Check sheet for the modelled part. Datum: model origin and axes. Units: mm. Face numbers are marked on the shaded views. A direction names the side the tool comes from. Round coordinates to 2 decimals unless told otherwise and drop trailing zeros. Write each loop counter-clockwise with the first axis right and the second up, starting at its lowest first coordinate (ties: lowest second). Pieces come first, ordered by that corner, then holes. Notation, with made-up numbers: M -33.75,89 L 18.25,89 A33 ccw 18.25,128 Z; hole C 32,24.5 d5. An arc over 180 degrees is marked long. One line per item, written item: value.
from build123d import *

# Parameters (mm, degrees)
ESQUISSE1_W        = 6
ESQUISSE1_H        = 55
BOSS_EXTRU_1_DEPTH = 3.5
ESQUISSE2_W        = 6
ESQUISSE2_H        = 2.5
BOSS_EXTRU_2_DEPTH = 35
ESQUISSE4_W        = 6
ESQUISSE4_H        = 2
BOSS_EXTRU_3_DEPTH = 15
ESQUISSE10_R       = 2.25
BOSS_EXTRU_4_DEPTH = 4.7
CONG_5_R           = 1


with BuildPart() as part:
    # Esquisse1 → Boss.-Extru.1 (new body)
    with BuildSketch(Plane.XY):
        with Locations((3, 27.5)):
            Rectangle(ESQUISSE1_W, ESQUISSE1_H)
    extrude(amount=BOSS_EXTRU_1_DEPTH)

    # Esquisse2 → Boss.-Extru.2 (add)
    with BuildSketch(Plane.XY.offset(3.5)):
        with Locations((3, 31.25)):
            Rectangle(ESQUISSE2_W, ESQUISSE2_H)
    extrude(amount=BOSS_EXTRU_2_DEPTH)

    # Esquisse4 → Boss.-Extru.3 (add)
    with BuildSketch(Plane(origin=(0, 30, 0), x_dir=(-1, 0, 0), z_dir=(0, -1, 0))):
        with Locations((-3, -37.5)):
            Rectangle(ESQUISSE4_W, ESQUISSE4_H)
    extrude(amount=BOSS_EXTRU_3_DEPTH)

    # Esquisse10 → Boss.-Extru.4 (add)
    with BuildSketch(Plane(origin=(0, 0, 36.5), x_dir=(-1, 0, 0), z_dir=(0, 0, -1))):
        with Locations(Location((-3, 18.95, 0), (0, 0, 180))):
            Circle(ESQUISSE10_R)
    extrude(amount=BOSS_EXTRU_4_DEPTH)

    # Congé5
    cong_5_edges = [part.edges().sort_by_distance(p)[0] for p in [
        (0.75, 18.95, 31.8),
    ]]
    fillet(cong_5_edges, radius=CONG_5_R)


solid = part.part
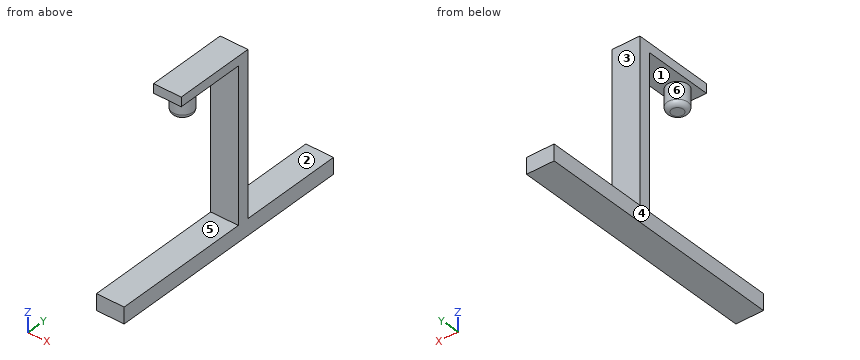
Q1. Sectioned sample at B-B on x = 3. Enter the section's corners in (y, z), and give its area (3 significant figures).
Completed:
outline: M 0,0 L 55,0 L 55,3.5 L 32.5,3.5 L 32.5,38.5 L 15,38.5 L 15,36.5 L 16.7,36.5 L 16.7,32.8 A1 ccw 17.7,31.8 L 20.2,31.8 A1 ccw 21.2,32.8 L 21.2,36.5 L 30,36.5 L 30,3.5 L 0,3.5 Z
area: 331 mm^2
Q2. Sectioned sample at A-A on y = 18.95. Enter the section's corners in (x, z).
Completed:
outline: M 0,0 L 6,0 L 6,3.5 L 0,3.5 Z; M 0,36.5 L 0.75,36.5 L 0.75,32.8 A1 ccw 1.75,31.8 L 4.25,31.8 A1 ccw 5.25,32.8 L 5.25,36.5 L 6,36.5 L 6,38.5 L 0,38.5 Z
Q3. Access from +Z, -Z, +X, -X, +Y, -Y to the whole of each face (thin tool, end or side, straight path). Record for the marked faces 4, 5 and 6.
Completed:
face 4: +Z, -Z, -X, +Y, -Y
face 5: +X, -X, -Y
face 6: none
Q4. Sectioned sample at D-D on y = 42.5. Enter the section's corners in (x, z), and give its area (3 significant figures).
Completed:
outline: M 0,0 L 6,0 L 6,3.5 L 0,3.5 Z
area: 21.0 mm^2
Q5. Sectioned sample at C-C on z = 34.5. Enter the section's corners in (x, y).
Completed:
outline: M 0,30 L 6,30 L 6,32.5 L 0,32.5 Z; C 3,18.95 d4.5
Q6. Depth check by flat-ended pin: P1, Ø1.5, axis at x = 3, y = 44, coming from the +Z side; P2, Ø1, axis at x = 5, z = 20.5, coming from the -Y side; P3, Ø2, axis at x = 3.5, z = 37, coming from the -Y side. Enter the tip coordinate at first touch or a pass-through.
Completed:
P1: z = 3.5
P2: y = 30
P3: y = 15
Q7. Scan lines: line 1 (Z direction, x = 1.25, y = 22); line 2 (Y direction, x = 0.95, z = 31); line 3 (Z direction, x = 3.85, y = 43). Record each from-to range of solid material in increasing order. Write a range as [from, to].
Completed:
line 1: [0, 3.5], [36.5, 38.5]
line 2: [30, 32.5]
line 3: [0, 3.5]
Q8. Draft check along Y on the marked faces 1, 2 and 3. Enter one of: pulls with the +Y half, pulls with the -Y half, needs draft (parallel to the pull), parting line crosses it, or undercut.
Completed:
face 1: undercut
face 2: needs draft
face 3: pulls with the +Y half
